Design review of the part built by this model. Coordinates are the model's own, in mm. A direction names the side the tool comes from. Coordinates: 2 decimals unless noted, no trailing zeros. Write each loop counter-clockwise with the first axis right and the second up, starting at its lowest first coordinate (ties: lowest second). Pieces come first, ordered by that corner, then holes. Notation, with made-up numbers: M -5.75,7.25 L 46.25,7.25 A7 cw 46.25,17.25 Z; hole C -12,76 d2. An arc over 180 degrees is marked long. One line per question, with ' | ' between items.
Autodesk Fusion 360 part; units mm, degrees
sketch "base plate" plane through (0, 0, 0) normal (0, 0, 1) x (1, 0, 0)
  line L0 (-20, 20) -> (20, 20)
  line L1 (20, 20) -> (20, -20)
  line L2 (20, -20) -> (-20, -20)
  line L3 (-20, -20) -> (-20, 20)
  line L4 (-20, 20) -> (20, -20) construction
  line L5 (20, 20) -> (-20, -20) construction
  dimension "d1" = 40
  dimension "d2" = 40
extrude "Extrude1" add sketch "base plate" along normal blind 5
sketch "holder" plane through (0, 0, 5) normal (0, 0, 1) x (-1, 0, 0)
  line L0 (20, 20) -> (-20, 20)
  line L1 (-20, 20) -> (-20, -20)
  line L2 (-20, -20) -> (20, -20)
  line L3 (20, -20) -> (20, 20)
  line L4 (20, 0) -> (-20, 0) construction
  line L5 (0, -20) -> (0, 20) construction
  circle A0 centre (0, 0) radius 5.525
  dimension "d5" = 11.05
extrude "Extrude2" add sketch "holder" along normal blind 2.5 contours A0
fillet "Fillet1" radius 1 6 faces at (0.1376, -15.1699, 5) (6.6667, -20, 3.3333) (20, 6.6667, 3.3333) (-6.6667, 6.6667, 0) (-6.6667, 20, 3.3333) (-20, -6.6667, 3.3333)
1. Tool access review of faces 1 (the face through (0.266, 19.699, 0.285)), 2 (the face through (-9, 0, 5)): name each direction out of +Z, -Z, +X, -X, +Y, -Y from which nothing blocks a thin tool from reaching the whole face with its end or side.
Answer sheet:
face 1: -Z, +X, -X, +Y | face 2: +Z
2. Take a section at B-B (x = 0). Write out the cut boundary in (y, z) (3 decimals), then the cut area to 3 significant figures.
Answer sheet:
outline: M -20,1 A1 ccw -19,0 L 19,0 A1 ccw 20,1 L 20,4 A1 ccw 19,5 L 6.525,5 A1 cw 5.525,6 L 5.525,7.5 L -5.525,7.5 L -5.525,6 A1 cw -6.525,5 L -19,5 A1 ccw -20,4 Z | area: 227 mm^2
3. Insertion check: pin 1 Ø8 at (x, y) = (-12, -7) entering from +Z. The pin has a flat end and moves straight along its axis. Give the tip position at first contact, or say it passes through.
Answer sheet:
pin 1: z = 5
4. To check wall thickness, follow line 1 along Y through (x, z) = (0, 6) (3 decimals); line 2 along Z through (x, y) = (-13.5, 7.5); line 3 along Y through (x, z) = (12, 0.5). State the ranges of each line that lie inside material, in increasing order. Write a range as [from, to].
Answer sheet:
line 1: [-5.525, 5.525] | line 2: [0, 5] | line 3: [-19.87, 19.87]
5. Take a section at A-A (y = -12.5). Write out the cut boundary in (x, z), then the cut area to 3 significant figures.
Answer sheet:
outline: M -20,1 A1 ccw -19,0 L 19,0 A1 ccw 20,1 L 20,4 A1 ccw 19,5 L -19,5 A1 ccw -20,4 Z | area: 199 mm^2
6. Take a section at C-C (z = 6.5). Write out the cut boundary in (x, y) (3 decimals), then the cut area to 3 significant figures.
Answer sheet:
outline: C 0,0 d11.05 | area: 95.9 mm^2
